```python
from build123d import *

# Parameters (mm, degrees)
SKETCH1_R                               = 150
BOSS_EXTRUDE2_DEPTH                     = 3
CBORE_FOR_M6_HEX_HEAD_BOLT1_D           = 6.6
CBORE_FOR_M6_HEX_HEAD_BOLT1_CBORE_D     = 14.55
CBORE_FOR_M6_HEX_HEAD_BOLT1_CBORE_DEPTH = 4.38


with BuildPart() as part:
    # Sketch1 → Boss-Extrude2 (new body)
    with BuildSketch(Plane.XY):
        Circle(SKETCH1_R)
    extrude(amount=BOSS_EXTRUDE2_DEPTH)

    # CBORE for M6 Hex Head Bolt1 (through all)
    with Locations(Plane(origin=(0, 0, 0), x_dir=(-1, 0, 0), z_dir=(0, 0, -1))):
        with Locations((-20.948618644, 13.643876902), (13.643876902, 20.948618644), (20.948618644, -13.643876902), (-13.643876902, -20.948618644)):
            CounterBoreHole(CBORE_FOR_M6_HEX_HEAD_BOLT1_D / 2, CBORE_FOR_M6_HEX_HEAD_BOLT1_CBORE_D / 2, CBORE_FOR_M6_HEX_HEAD_BOLT1_CBORE_DEPTH)


solid = part.part
```
Build history of the part. All positions in model axes, mm. Coordinates: 2 decimals unless noted, no trailing zeros. Order: outer loops, then holes, each group sorted by start corner. A loop starts at its lowest first (then second) coordinate and runs counter-clockwise, first axis right, second up. Notation, with made-up numbers: (51, 69) -> (84, 69) arc R33 ccw to (84, 101) -> close; hole circle Ø7 at (67, -2). An arc over 180 degrees is marked (long way). Answer in a Markdown table with one row per item. Add a question column.
Q1. Band-saw the part on C-C, the plane x = 108.5. List the corners of the cut face in (y, z).
Q2. Band-saw the part on A-A, the plane z = 0.5. List the corners of the cut face in (x, y) (3 decimals), then the cut area to 3 significant figures.
Q3. Drop flat-ended pins along their axis: pin 1 (11.5 mm diameter, centred on x = 13.64, y = -20.95, fed in from -Z); pin 2 (23.5 mm diameter, centred on x = 20.95, y = 13.64, fed in from +Z); pin 3 (1 mm diameter, centred on x = -98, z = 1, fed in from +Y). Give the stop position or say it passes through.
Q4. Band-saw the part on B-B, the plane y = 111. List the corners of the cut face in (x, z), then the cut area to 3 significant figures.
Q5. Wall check: line 1 along Y through (x, z) = (18.5, 2.65); line 2 along X through (y, z) = (12.5, 2.2); line 3 along X through (y, z) = (29.5, 2.35). Give the ranges that are in metal, low to high. Write a range as [from, to].
Q6. Mould opens along Y. For faces 1 (the face through (26.722, 9.217, 1.479)), 2 (the face through (-2, 2, 3)), 3 (the face through (-17.001, 14.494, 1.479)), 4 (the face through (-19.527, 148.724, 1.479)) say: +Y half, -Y half, draft (parallel to the pull), parting line (faces both ways), or undercut.
Answers follow:
| question | item | result |
|---|---|---|
| 1 | outline | (-103.57, 0) -> (103.57, 0) -> (103.57, 3) -> (-103.57, 3) -> close |
| 2 | outline | circle Ø300 at (0, 0); hole circle Ø14.55 at (-20.949, -13.644); hole circle Ø14.55 at (-13.644, 20.949); hole circle Ø14.55 at (13.644, -20.949); hole circle Ø14.55 at (20.949, 13.644) |
| 2 | area | 70,000 mm^2 |
| 3 | pin 1 | through |
| 3 | pin 2 | z = 3 |
| 3 | pin 3 | y = 113.99 |
| 4 | outline | (-100.89, 0) -> (100.89, 0) -> (100.89, 3) -> (-100.89, 3) -> close |
| 4 | area | 605 mm^2 |
| 5 | line 1 | [-148.85, -26.37], [-15.53, 6.79], [20.49, 148.85] |
| 5 | line 2 | [-149.48, 13.76], [28.13, 149.48] |
| 5 | line 3 | [-147.07, 147.07] |
| 6 | face 1 | undercut |
| 6 | face 2 | draft |
| 6 | face 3 | undercut |
| 6 | face 4 | parting line |
